from build123d import *

# Parameters (mm, degrees)
F0_W            = 305
F0_H            = 200
F1_DEPTH        = 25
F3_D            = 8.5
F5_DEPTH        = 152.501
F5_DEPTH_BACK   = 152.501
F6_SIZE         = 1
F10_D           = 6.35
F10_DEPTH       = 42
F10_TIP         = 1.9077324654
F11_D           = 6.35
F11_DEPTH       = 57
F11_TIP         = 1.9077324654
F11_ON_F8_D     = 6.35
F11_ON_F8_DEPTH = 57
F11_ON_F8_TIP   = 1.9077324654


with BuildPart() as f1:
    # F0 (on Top) → F1 (new body)
    with BuildSketch(Plane.XY):
        Rectangle(F0_W, F0_H)
    extrude(amount=-F1_DEPTH)

    # F3 (through all)
    with Locations(Plane.XY):
        with Locations((-137.5, 75), (137.5, 75), (137.5, -75), (-137.5, -75)):
            Hole(F3_D / 2)

    # F4 (on Right) → F5 (cut, two sides)
    with BuildSketch(Plane.YZ) as f5_sk:
        Polygon((-34.75, 0), (-40, 0), (-45.25, 0), (-45.25, -6.5), (-48.25, -6.5), (-48.25, -13.5), (-40, -13.5), (-31.75, -13.5), (-31.75, -6.5), (-34.75, -6.5), align=None)
        Polygon((65.25, 0), (60, 0), (54.75, 0), (54.75, -6.5), (51.75, -6.5), (51.75, -13.5), (60, -13.5), (68.25, -13.5), (68.25, -6.5), (65.25, -6.5), align=None)
    extrude(amount=-F5_DEPTH, mode=Mode.SUBTRACT)
    extrude(f5_sk.sketch, amount=F5_DEPTH_BACK, mode=Mode.SUBTRACT)

    # F6
    f6_edges = [f1.edges().sort_by_distance(p)[0] for p in [
        (0, -34.75, 0),
        (0, -45.25, 0),
        (0, 65.25, 0),
        (0, 54.75, 0),
    ]]
    chamfer(f6_edges, length=F6_SIZE)

    # F10
    with Locations(Plane.XZ.offset(100)):
        with Locations((97.5, -12.5), (-97.5, -12.5)):
            Hole(F10_D / 2, depth=F10_DEPTH)
            with Locations((0, 0, -(F10_DEPTH + F10_TIP / 2))):  # 118° drill point
                Cone(0, F10_D / 2, F10_TIP, mode=Mode.SUBTRACT)

    # F11
    with Locations(Plane(origin=(-152.5, 0, 0), x_dir=(0, -1, 0), z_dir=(-1, 0, 0))):
        with Locations((60, -12.5)):
            Hole(F11_D / 2, depth=F11_DEPTH)
            with Locations((0, 0, -(F11_DEPTH + F11_TIP / 2))):  # 118° drill point
                Cone(0, F11_D / 2, F11_TIP, mode=Mode.SUBTRACT)

    # F11 on F8
    with Locations(Plane.YZ.offset(152.5)):
        with Locations((-60, -12.5)):
            Hole(F11_ON_F8_D / 2, depth=F11_ON_F8_DEPTH)
            with Locations((0, 0, -(F11_ON_F8_DEPTH + F11_ON_F8_TIP / 2))):  # 118° drill point
                Cone(0, F11_ON_F8_D / 2, F11_ON_F8_TIP, mode=Mode.SUBTRACT)


solid = f1.part
Geometry check sheet. Reference: the model listing, model coordinates, mm. A direction names the side the tool comes from. Give positions to 0.01 mm unless a question says otherwise; leave off trailing zeros. Write each loop counter-clockwise with the first axis right and the second up, starting at its lowest first coordinate (ties: lowest second). Pieces come first, ordered by that corner, then holes.
1) Go/stop test with a flat-tipped pin: pin 1 Ø5 at (x, y) = (-63, 58) entering from +Z. Record where the tip stops, or that it passes through.
Values follow:
pin 1: stops at z = -13.5
2) Set-up check for faces 1 (the face through (124.62, -56.83, -12.36)), 2 (the face through (2, 51.75, -10)), 3 (the face through (2, 65.25, -4)), 4 (the face through (-94.33, -79.72, -12.36)): record each of +Z, -Z, +X, -X, +Y, -Y from which the full face is reachable in a straight line by a thin tool's end or side.
Values follow:
face 1: +X
face 2: +X, -X
face 3: +Z, +X, -X
face 4: -Y
3) Cross-section at B-B (x = -137.5). Count the separate pieces of the cut face and the enclosed holes in it, plus the area to 3 significant figures.
Values follow:
separate pieces: 3
enclosed holes: 1
area: 4,170 mm2
4) Cross-section at C-C (y = 75). Record the boundary of the cut face in (x, z).
Values follow:
outline: (-152.5, -25) - (-141.75, -25) - (-141.75, 0) - (-152.5, 0) - close; (-133.25, -25) - (133.25, -25) - (133.25, 0) - (-133.25, 0) - close; (141.75, -25) - (152.5, -25) - (152.5, 0) - (141.75, 0) - close
5) Cross-section at A-A (y = -75). Record the boundary of the cut face in (x, z) (3 decimals), plus the area to 3 significant figures.
Values follow:
outline: (-152.5, -25) - (-141.75, -25) - (-141.75, 0) - (-152.5, 0) - close; (-133.25, -25) - (133.25, -25) - (133.25, 0) - (-133.25, 0) - close; (141.75, -25) - (152.5, -25) - (152.5, 0) - (141.75, 0) - close; hole circle Ø6.35 at (-97.5, -12.5); hole circle Ø6.35 at (97.5, -12.5)
area: 7,140 mm2
6) Cross-section at D-D (x = 108). Record the boundary of the cut face in (y, z) (3 decimals), plus the area to 3 significant figures.
Values follow:
outline: (-100, -25) - (100, -25) - (100, 0) - (66.25, 0) - (65.25, -1) - (65.25, -6.5) - (68.25, -6.5) - (68.25, -13.5) - (51.75, -13.5) - (51.75, -6.5) - (54.75, -6.5) - (54.75, -1) - (53.75, 0) - (-33.75, 0) - (-34.75, -1) - (-34.75, -6.5) - (-31.75, -6.5) - (-31.75, -13.5) - (-48.25, -13.5) - (-48.25, -6.5) - (-45.25, -6.5) - (-45.25, -1) - (-46.25, 0) - (-100, 0) - close; hole circle Ø6.35 at (-60, -12.5)
area: 4,600 mm2
7) Release check for a two-part mould opening along X. For faces 5 (the face through (-152.5, -1, -12)), 6 (the face through (140.87, 72.41, -12.68)), 7 (the face through (-2, 11, 0)) record: released by +X, released by -X, zero draft, split by the parting line, or undercut.
Values follow:
face 5: released by -X
face 6: undercut
face 7: zero draft
8) Thickness scan on line 1 (Y direction, x = 33, z = -12.5); line 2 (Y direction, x = -29.5, z = -3); line 3 (Y direction, x = -121, z = -12.5) (3 decimals). Record the ranges inside material, lowest first.
Values follow:
line 1: y = -100 to -48.25, -31.75 to 51.75, 68.25 to 100
line 2: y = -100 to -45.25, -34.75 to 54.75, 65.25 to 100
line 3: y = -100 to -63.175, -56.825 to -48.25, -31.75 to 51.75, 68.25 to 100
